Here's how the part is built. I have some questions about the finished solid (model axes, mm). A direction names the side the tool comes from. Coordinates: 2 decimals unless noted, no trailing zeros. Loops run counter-clockwise (first coordinate to the right, second up) from the corner with the lowest first, then second, coordinate; pieces in that order, holes last. Notation, with made-up numbers: (2.25, 5.25) -> (41.25, 5.25) arc R17 cw to (41.25, 38.25) -> close; hole circle Ø9 at (-6.5, 51.25). An arc over 180 degrees is marked (long way). Answer as a JSON object with one key per item and string values. Group by question number.
1) I need wall thicknesses on probe 1 along Z at (x, y) = (-560, 452); probe 2 along Z at (x, y) = (-449, 390); probe 3 along Y at (x, z) = (-569, 366.5). Which ranges of each line are inside material? Lowest first, please. Write a range as [from, to].
2) I'm going to push flat-ended pins straight in: pin 1 (25 mm diameter, centred on y = 440, z = -84.5, fed in from +X); pin 2 (15 mm diameter, centred on x = -555.5, z = 122.5, fed in from -Y); pin 3 (15 mm diameter, centred on y = 488, z = 115, fed in from -X); pin 4 (10 mm diameter, centred on x = -514.5, z = -29, fed in from +Y). Where does each tip first touch, or does it pass through?
3) If we mould it in two halves opening along Z, with no side actions, what happens to faces 1 (the cylindrical face through (-401.91, 429.05, 394.3)), 2 (the flat face through (-546, 453, 182)), 3 (the flat face through (-546, 403, -95)), 4 (the flat face through (-546, 428, -70))? For each: +Z half, -Z half, draft (parallel to the pull), parting line (faces both ways), or undercut.
4) Which directions (+Z, -Z, +X, -X, +Y, -Y) give clear straight access to the entire face, cutting with the end or side of a thin tool? Please do faces 5 (the flat face through (-520.892, 478, 126)), 6 (the flat face through (-534, 503, 177)), 7 (the flat face through (-570.892, 428, -95)).
5) I want a section at D-D (z = 248.5). Write out the boundary of the cut face in (x, y), then the cut area to 3 significant figures.
Autodesk Inventor part; units mm, degrees
ref_plane "YZ Plane" through (0, 0, 0) normal (1, 0, 0) x (0, 1, 0)
ref_plane "XZ Plane" through (0, 0, 0) normal (0, 1, 0) x (-1, 0, 0)
ref_plane "XY Plane" through (0, 0, 0) normal (0, 0, 1) x (1, 0, 0)
ref_plane "Work Plane1" through (-0.3785, 403, -180) normal (0, 1, 0) x (-1, 0, 0)
sketch "Sketch1" plane through (-0.3785, 403, -180) normal (0, 1, 0) x (-1, 0, 0)
  line L0 (545.5132, 110) -> (570.5132, 110)
  line L1 (570.5132, 110) -> (570.5132, 60)
  line L2 (570.5132, 60) -> (545.5132, 60)
  line L3 (545.5132, 60) -> (520.5132, 60)
  line L4 (520.5132, 60) -> (520.5132, 110)
  line L5 (520.5132, 110) -> (545.5132, 110)
  point P0 (-0.3785, 180)
  dimension "d2" = 25
  dimension "d3" = 25
extrude "Extrusion1" add sketch "Sketch1" along normal blind 50
sketch "Sketch2" plane through (-520.8916, 403, -120) normal (0, 0, -1) x (-1, 0, 0)
  line L0 (50, 50) -> (0, 50)
  line L1 (50, 50) -> (0, 50)
  line L2 (0, 50) -> (0, 100)
  line L3 (0, 100) -> (50, 100)
  line L4 (50, 100) -> (50, 50)
  point P0 (-520.8916, -403)
  dimension "d6" = 50
extrude "Extrusion2" add sketch "Sketch2" against normal blind 500
sketch "Sketch3" plane through (-520.8916, 403, 380) normal (0, 0, 1) x (1, 0, 0)
  line L0 (0, 100) -> (-50, 100)
  line L1 (-50, 100) -> (-50, 50)
  line L2 (-50, 50) -> (0, 50)
  line L3 (0, 50) -> (0, 100)
  line L4 (-25, 100) -> (125, 100)
  line L5 (125, 100) -> (-175, 100)
  line L6 (-175, 100) -> (-175, -50)
  line L7 (-175, -50) -> (125, -50)
  line L8 (125, -50) -> (125, 100)
  point P0 (520.8916, -403)
  dimension "d9" = 150
  dimension "d10" = 300
  dimension "d11" = 150
extrude "Extrusion3" add sketch "Sketch3" along normal blind 20
fillet "Fillet1" radius 20 3 edges at (-695.8916, 428, 400) (-545.8916, 353, 400) (-395.8916, 428, 400)
Determined:
{
 "1": {"probe 1": "[-120, -70], [380, 400]", "probe 2": "[380, 400]", "probe 3": "[453, 503]"},
 "2": {"pin 1": "x = -520.89", "pin 2": "y = 453", "pin 3": "x = -570.89", "pin 4": "through"},
 "3": {"face 1": "+Z half", "face 2": "undercut", "face 3": "draft", "face 4": "undercut"},
 "4": {"face 5": "-Z, +X, +Y, -Y", "face 6": "+Z, -Z, +X, -X, +Y", "face 7": "-Z, -X, +Y, -Y"},
 "5": {"outline": "(-570.89, 453) -> (-520.89, 453) -> (-520.89, 503) -> (-570.89, 503) -> close", "area": "2,500 mm^2"}
}
